Check sheet for the modelled part. Datum: model origin and axes. Units: mm. Round coordinates to 2 decimals unless told otherwise and drop trailing zeros. Write each loop counter-clockwise with the first axis right and the second up, starting at its lowest first coordinate (ties: lowest second). Pieces come first, ordered by that corner, then holes. Notation, with made-up numbers: (-24.75, 67.5) - (-18.75, 67.5) arc R18 cw to (-18.75, 77.5) - close; hole circle Ø4 at (13, -14). An arc over 180 degrees is marked (long way). Use one line per item in the form item = value. Start each with the question number.
1) Draft check along Z on faces 1 (the face through (-110.9, 1.5, -17)), 2 (the face through (-49.635, 1.479, -48.348)), 3 (the face through (-58, 3, -58)). Enter one of: +Z half, -Z half, draft (parallel to the pull), parting line (faces both ways), or undercut.
2) Section check A-A (y = 32). Record the boundary of the cut face in (x, z).
3) Scan lines: probe 1 along Y at (x, z) = (-31.5, -86); probe 2 along Z at (x, y) = (-131, 11); probe 3 along X at (y, z) = (31, -73.5). Record each from-to range of solid material in increasing order.
4) Section check B-B (y = 14). Record the boundary of the cut face in (x, z).
5) Section check C-C (x = -134). Record the boundary of the cut face in (y, z), then the cut area to 3 significant figures.
6) Gauge pin test, flat ends, axial feed: P1, Ø1.5, axis at y = 13.5, z = -57, coming from the -X side; P2, Ø6, axis at y = 14, z = -116, coming from the -X side; P3, Ø8, axis at x = -108.03, z = -16.11, coming from the +Y side. Record the tip position at first contact, or that the pin passes through.
Autodesk Inventor part; units mm, degrees
ref_plane "YZ Plane" through (0, 0, 0) normal (1, 0, 0) x (0, 1, 0)
ref_plane "XZ Plane" through (0, 0, 0) normal (0, 1, 0) x (-1, 0, 0)
ref_plane "XY Plane" through (0, 0, 0) normal (0, 0, 1) x (1, 0, 0)
sketch "Sketch1" plane through (0, 0, 0) normal (0, 1, 0) x (-1, 0, 0)
  line L0 (0, 0) -> (0, -650)
  line L1 (0, -650) -> (650, -650)
  line L2 (650, -650) -> (650, 0)
  line L3 (650, 0) -> (0, 0)
  line L4 (0, 0) -> (3, 0)
  line L5 (3, 0) -> (3, -650)
  line L6 (3, -650) -> (0, -650)
  line L7 (0, -650) -> (0, -647)
  line L8 (0, -647) -> (650, -647)
  line L9 (650, -647) -> (650, -650)
  line L10 (650, -650) -> (647, -650)
  line L11 (647, -650) -> (647, 0)
  line L12 (647, 0) -> (650, 0)
  line L13 (650, 0) -> (650, -3)
  line L14 (650, -3) -> (0, -3)
  line L15 (0, -3) -> (0, 0)
  line L16 (0, 0) -> (0, -37)
  line L17 (0, -37) -> (650, -37)
  line L18 (650, -37) -> (650, 0)
  line L19 (650, 0) -> (613, 0)
  line L20 (613, 0) -> (613, -650)
  line L21 (613, -650) -> (650, -650)
  line L22 (650, -650) -> (650, -613)
  line L23 (650, -613) -> (0, -613)
  line L24 (0, -613) -> (0, -650)
  line L25 (0, -650) -> (37, -650)
  line L26 (37, -650) -> (37, 0)
  line L27 (37, 0) -> (0, 0)
  line L28 (0, 0) -> (650, -650)
  line L29 (650, 0) -> (0, -650)
  line L30 (37, -3) -> (3, -37)
  line L31 (20, -20) -> (75.1543, -75.1543)
  line L32 (75.1543, -75.1543) -> (3, -147.3087)
  line L33 (75.1543, -75.1543) -> (147.3087, -3)
  line L34 (75.1543, -75.1543) -> (48.9914, -48.9914)
  line L35 (48.9914, -48.9914) -> (3, -94.9828)
  line L36 (48.9914, -48.9914) -> (94.9828, -3)
  line L37 (75.1543, -75.1543) -> (77.2756, -77.2756)
  line L38 (77.2756, -77.2756) -> (3, -151.5513)
  line L39 (77.2756, -77.2756) -> (151.5513, -3)
  line L40 (75.1543, -75.1543) -> (68.0833, -68.0833)
  line L41 (68.0833, -68.0833) -> (57.8302, -78.3363)
  line L42 (68.0833, -68.0833) -> (78.3363, -57.8302)
  circle A0 centre (78.3363, -57.8302) radius 1.5
  circle A1 centre (57.8302, -78.3363) radius 1.5
  line L43 (3, -147.3087) -> (3, -94.9828)
  line L44 (147.3087, -3) -> (94.9828, -3)
  line L45 (121.1457, -3) -> (3, -121.1457)
  circle A2 centre (62.0729, -62.0729) radius 65
  circle A3 centre (108.0348, -16.1109) radius 3
  circle A4 centre (16.1109, -108.0348) radius 3
  dimension "d0" = 650
  dimension "d1" = 650
  dimension "d2" = 650
  dimension "d3" = 3
  dimension "d4" = 650
  dimension "d5" = 3
  dimension "d6" = 3
  dimension "d7" = 650
  dimension "d8" = 3
  dimension "d9" = 650
  dimension "d10" = 37
  dimension "d11" = 650
  dimension "d12" = 37
  dimension "d13" = 650
  dimension "d14" = 37
  dimension "d15" = 650
  dimension "d16" = 37
  dimension "d17" = 650
  dimension "d18" = 78
  dimension "d19" = 37
  dimension "d20" = 3
  dimension "d21" = 10
  dimension "d22" = 14.5
  dimension "d23" = 14.5
  dimension "d24" = 3
  dimension "d25" = 3
  dimension "d26" = 130
  dimension "d27" = 6
  dimension "d28" = 6
extrude "Extrusion1" add sketch "Sketch1" along normal blind 3 contours L35 A2 A4 L45 L5 | L35 L26 L45 A4 A2 | L36 A2 A3 L45 L17 | L17 L45 L28 L36 | L35 L28 L45 L26 | L14 L45 A3 A2 L36 | L45 A4 A2 L32 L5 | L45 A3 A2 L33 L17 | L17 L33 L28 L45 | L45 L28 L32 L26 | L26 L32 A2 A4 L45 | L14 L33 A2 A3 L45
extrude "Extrusion2" add sketch "Sketch1" along normal blind 37 contours L5 L32 A2 L38 | L39 A2 L33 L14 | L33 A2 L39 L17 | L17 L39 L28 L33 | L32 L28 L38 L26 | L26 L38 A2 L32
sketch "Sketch2" plane through (-151.5513, 0, -3) normal (-0.7071, 0, -0.7071) x (-0.7071, 0, 0.7071)
  line L0 (-105.0416, 0) -> (-105.0416, 3)
  line L1 (-105.0416, 3) -> (-105.0416, 23)
  line L2 (-3, 37) -> (-207.0833, 37)
  line L3 (-105.0416, 23) -> (-105.0416, 16)
  circle A0 centre (-105.0416, 16) radius 6
  dimension "d33" = 3
  dimension "d39" = 20
  dimension "d40" = 7
  dimension "d41" = 12
extrude "Extrusion4" cut sketch "Sketch2" against normal blind 10
properties part number "body_inner_L_clamp"
Results are:
q1.face_1 = undercut
q1.face_2 = +Z half
q1.face_3 = draft
q2.outline = (-151.55, -3) - (-77.28, -77.28) - (-3, -151.55) - (-3, -147.31) - (-75.15, -75.15) - (-147.31, -3) - close
q3.probe_1 = 0 to 3
q3.probe_2 = -23.55 to -19.31
q3.probe_3 = -81.05 to -76.81
q4.outline = (-151.55, -3) - (-81.28, -73.28) - (-79.15, -71.15) - (-147.31, -3) - close; (-73.28, -81.28) - (-3, -151.55) - (-3, -147.31) - (-71.15, -79.15) - close
q5.outline = (0, -20.55) - (37, -20.55) - (37, -16.31) - (3, -16.31) - (3, -3) - (0, -3) - close
q5.area = 197 mm²
q6.P1 = -98.3
q6.P2 = -41.55
q6.P3 = 3
